from build123d import *

# Parameters (mm, degrees)
SKETCH003_R      = 1.5
EXTRUDE003_DEPTH = 1.5
EXTRUDE002_DEPTH = 3
SKETCH001_W      = 25
SKETCH001_H      = 12
EXTRUDE001_DEPTH = 1.5
EXTRUDE_DEPTH    = 3
FILLET_R         = 2
FILLET001_R      = 3
FILLET002_R      = 3


with BuildPart() as extrude003:
    # Sketch003 (on Face18 of Fillet002) → Extrude003 (new body)
    with BuildSketch(Plane.XY.offset(1.5)):
        with Locations((-6.5, 1)):
            Circle(SKETCH003_R)
        with Locations((6.5, 1)):
            Circle(SKETCH003_R)
    extrude(amount=-EXTRUDE003_DEPTH)


with BuildPart() as extrude002:
    # Sketch002 (on Face8 of Cut) → Extrude002 (new body)
    with BuildSketch(Plane.XY.offset(3)):
        Polygon((0, 22), (-9.5, 10), (9.5, 10), align=None)
    extrude(amount=-EXTRUDE002_DEPTH)


with BuildPart() as extrude001:
    # Sketch001 (on Face7 of Extrude) → Extrude001 (new body)
    with BuildSketch(Plane.XY.offset(3)):
        with Locations((0, 1)):
            Rectangle(SKETCH001_W, SKETCH001_H)
    extrude(amount=-EXTRUDE001_DEPTH)


with BuildPart() as cut002:
    # Sketch → Extrude (new body)
    with BuildSketch(Plane.XY):
        Polygon((-12.5, -5), (12.5, -5), (12.5, 10), (0, 25), (-12.5, 10), align=None)
    extrude(amount=EXTRUDE_DEPTH)

    # Cut: cut Extrude001
    add(extrude001.part, mode=Mode.SUBTRACT)

    # Cut001: cut Extrude002
    add(extrude002.part, mode=Mode.SUBTRACT)

    # Fillet
    fillet_edges = [cut002.edges().sort_by_distance(p)[0] for p in [
        (0, 22, 1.5),
        (-9.5, 10, 1.5),
        (9.5, 10, 1.5),
    ]]
    fillet(fillet_edges, radius=FILLET_R)

    # Fillet001
    fillet001_edges = [cut002.edges().sort_by_distance(p)[0] for p in [
        (-12.5, 10, 1.5),
        (12.5, 10, 1.5),
        (0, 25, 1.5),
    ]]
    fillet(fillet001_edges, radius=FILLET001_R)

    # Fillet002
    fillet002_edges = [cut002.edges().sort_by_distance(p)[0] for p in [
        (12.5, -5, 0.75),
        (-12.5, -5, 0.75),
    ]]
    fillet(fillet002_edges, radius=FILLET002_R)

    # Cut002: cut Extrude003
    add(extrude003.part, mode=Mode.SUBTRACT)


solid = cut002.part
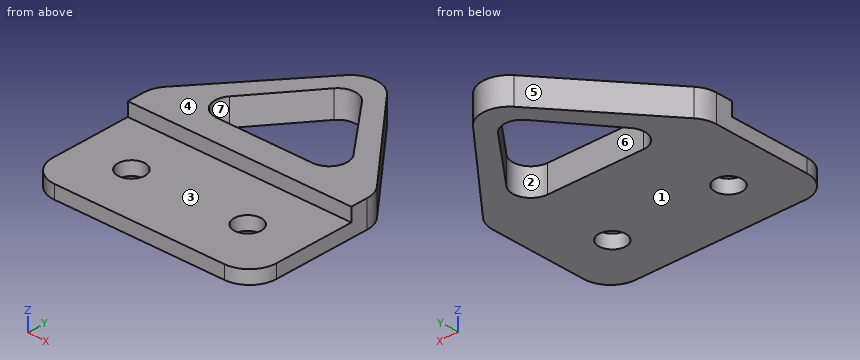
Model file for the job. Use its own axes, mm. Face numbers are marked on the shaded views. A direction names the side the tool comes from. Give positions to 0.01 mm unless a question says otherwise; leave off trailing zeros. Loops run counter-clockwise (first coordinate to the right, second up) from the corner with the lowest first, then second, coordinate; pieces in that order, holes last.
1) Tool access for the marked faces 1, 2 and 3: list every direction of +Z, -Z, +X, -X, +Y, -Y with a clear straight run to the whole face (end or side of a thin tool).
2) Flat gauge pins, fed straight in: pin 1 Ø10 at (x, y) = (-2, 11.5) entering from -Z; pin 2 Ø9.5 at (x, y) = (-5, 0) entering from +Z; pin 3 Ø1.2 at (x, z) = (3.5, 2.5) entering from -Y. Where does each tip first touch, or does it go through?
3) Pull direction Y, two halves, no side cores. Call the marked faces 4, 5, 6 and 7: +Y half, -Y half, draft (parallel to the pull), parting line (faces both ways), or undercut.
4) Saw through at A-A (y = 16). Write the cut outline in (x, z), plus the area to 3 significant figures.
5) Saw through at B-B (z = 2.4). Write the cut outline in (x, y).
6) Saw through at C-C (x = 6.5). Write the cut outline in (y, z).
7) Wall check: line 1 (Y direction, x = -6.5, z = 0.6); line 2 (Z direction, x = -0.75, y = -1.5); line 3 (X direction, y = 17.75, z = 1.25). Give the ranges that are in metal, low to high.
8) Saw through at D-D (y = 1). Write the cut outline in (x, z).
Answer block:
1. face 1: -Z, +X, -X, +Y, -Y
1. face 2: +Z, -Z
1. face 3: +Z, +X, -X, -Y
2. pin 1: stops at z = 0
2. pin 2: stops at z = 1.5
2. pin 3: stops at y = 7
3. face 4: draft
3. face 5: +Y half
3. face 6: undercut
3. face 7: undercut
4. outline: (-7.5, 0) - (-4.75, 0) - (-4.75, 3) - (-7.5, 3) - close; (4.75, 0) - (7.5, 0) - (7.5, 3) - (4.75, 3) - close
4. area: 16.5 mm2
5. outline: (-12.5, 7) - (12.5, 7) - (12.5, 8.91) arc R3 ccw to (11.8, 10.83) - (2.3, 22.23) arc R3 ccw to (-2.3, 22.23) - (-11.8, 10.83) arc R3 ccw to (-12.5, 8.91) - close; hole (-6.93, 13.24) arc R2 ccw to (-5.37, 10) - (5.37, 10) arc R2 ccw to (6.93, 13.24) - (1.57, 20.02) arc R2 ccw to (-1.57, 20.02) - close
6. outline: (-5, 0) - (-0.5, 0) - (-0.5, 1.5) - (-5, 1.5) - close; (2.5, 0) - (10.35, 0) - (10.35, 3) - (7, 3) - (7, 1.5) - (2.5, 1.5) - close; (13.79, 0) - (17.2, 0) - (17.2, 3) - (13.79, 3) - close
7. line 1: y = -5 to -0.5, 2.5 to 10.35, 13.79 to 17.2
7. line 2: z = 0 to 1.5
7. line 3: x = -6.04 to -3.36, 3.36 to 6.04
8. outline: (-12.5, 0) - (-8, 0) - (-8, 1.5) - (-12.5, 1.5) - close; (-5, 0) - (5, 0) - (5, 1.5) - (-5, 1.5) - close; (8, 0) - (12.5, 0) - (12.5, 1.5) - (8, 1.5) - close
